The model under review builds one solid part; all positions refer to its coordinate system, in mm. Coordinates: 2 decimals unless noted, no trailing zeros. Loops run counter-clockwise (first coordinate to the right, second up) from the corner with the lowest first, then second, coordinate; pieces in that order, holes last. Notation, with made-up numbers: M 71.5,30 L 104.5,30 A18 ccw 104.5,56 Z; hole C 51,78 d11. An arc over 180 degrees is marked long. Return JSON: item names as keys, results as strings.
```python
from build123d import *

# Parameters (mm, degrees)
SKETCH1_R           = 175
BOSS_EXTRUDE2_DEPTH = 10
SKETCH2_R           = 6
CUT_EXTRUDE1_DEPTH  = 248.68932153
CIRPATTERN2_COUNT   = 6


with BuildPart() as part:
    # Sketch1 → Boss-Extrude2 (new body)
    with BuildSketch(Plane.XY):
        Circle(SKETCH1_R)
        with BuildLine():
            ThreePointArc((30.001118034, 0.000363271), (24.271455118, -17.633432061), (9.271068846, -28.531513848))
            ThreePointArc((9.271068846, -28.531513848), (-9.270509831, -28.531695489), (-24.270855318, -17.633082037))
            ThreePointArc((-24.270855318, -17.633082037), (-30.000690983, 0.000951057), (-24.270855318, 17.63498415))
            ThreePointArc((-24.270855318, 17.63498415), (-9.270509831, 28.533597602), (9.271068846, 28.533415961))
            ThreePointArc((9.271068846, 28.533415961), (24.271455118, 17.635334174), (30.001118034, 0.001538842))
            ThreePointArc((30.001118034, 0.001538842), (30.001118028, 0.000951057), (30.001118011, 0.000363271))
        make_face(mode=Mode.SUBTRACT)
    extrude(amount=BOSS_EXTRUDE2_DEPTH)

    # Sketch2 → Cut-Extrude1 (cut, through all)
    with BuildSketch(Plane(origin=(0, 0, 0), x_dir=(-1, 0, 0), z_dir=(0, 0, -1))):
        with Locations((0, 70)):
            Circle(SKETCH2_R)
        with Locations((0, 150)):
            Circle(SKETCH2_R)
    cut_extrude1 = extrude(amount=-CUT_EXTRUDE1_DEPTH, mode=Mode.SUBTRACT)

    # CirPattern2: Cut-Extrude1 ×6 about axis
    cirpattern2_axis = Axis((0, 0, 0), (0, 0, 1))
    for i in range(1, CIRPATTERN2_COUNT):
        add(cut_extrude1.rotate(cirpattern2_axis, i * 360 / CIRPATTERN2_COUNT), mode=Mode.SUBTRACT)


solid = part.part
```
1. Add section D-D on z = 7.5. State how many separate pieces and enclosed holes the cut face has, plus the area to 3 significant figures.
Check values:
{"separate pieces": "1", "enclosed holes": "13", "area": "92,000 mm²"}
2. To check wall thickness, follow line 1 (Y direction, x = 0, z = 5.75); line 2 (X direction, y = -37.5, z = 1.5); line 3 (Y direction, x = -127, z = 6.5). State the ranges of each line that lie inside material, in increasing order.
Check values:
{"line 1": "-175 to -156, -144 to -76, -64 to -30, 30 to 64, 76 to 144, 156 to 175", "line 2": "-170.93 to -66.08, -55.17 to 55.17, 66.08 to 170.93", "line 3": "-120.4 to -80.25, -69.75 to 69.75, 80.25 to 120.4"}
3. Add section A-A on x = 0. Give the boundary of the cut face in (y, z).
Check values:
{"outline": "M -175,0 L -156,0 L -156,10 L -175,10 Z; M -144,0 L -76,0 L -76,10 L -144,10 Z; M -64,0 L -30,0 L -30,10 L -64,10 Z; M 30,0 L 64,0 L 64,10 L 30,10 Z; M 76,0 L 144,0 L 144,10 L 76,10 Z; M 156,0 L 175,0 L 175,10 L 156,10 Z"}
4. Add section C-C on y = 35. Give the boundary of the cut face in (x, z), plus the area to 3 significant figures.
Check values:
{"outline": "M -171.46,0 L -66.62,0 L -66.62,10 L -171.46,10 Z; M -54.62,0 L 54.62,0 L 54.62,10 L -54.62,10 Z; M 66.62,0 L 171.46,0 L 171.46,10 L 66.62,10 Z", "area": "3,190 mm²"}
5. Insertion check: pin 1 Ø11 at (x, y) = (129.9, 75) entering from +Z; pin 2 Ø3 at (y, z) = (57.5, 8) entering from +X; pin 3 Ø2 at (y, z) = (46, 1.5) entering from -X. Each pin has a flat end and moves straight along its axis. Give the tip position at first contact, or say it passes through.
Check values:
{"pin 1": "through", "pin 2": "x = 165.8", "pin 3": "x = -169.12"}
6. The part is to be moulded in two halves that separate along Y. For faces 1 (the face through (-124.18, 73.2, 4.93)), 2 (the face through (36, 2, 0)), 3 (the face through (-128.982, 118.273, 4.93)), say which applies: released by +Y, released by -Y, zero draft, split by the parting line, or undercut.
Check values:
{"face 1": "undercut", "face 2": "zero draft", "face 3": "split by the parting line"}
7. Add section B-B on y = -150. Give the boundary of the cut face in (x, z).
Check values:
{"outline": "M -90.14,0 L -6,0 L -6,10 L -90.14,10 Z; M 6,0 L 90.14,0 L 90.14,10 L 6,10 Z"}
